```python
from build123d import *

# Parameters (mm, degrees)
F2_R     = 7.62
F3_DEPTH = 76.2


with BuildPart() as f1:
    # F0 (on Front) → F1 (revolve)
    with BuildSketch(Plane.XZ):
        with BuildLine():
            Line((0, -25.4), (0, 25.4))
            ThreePointArc((0, 25.4), (-25.4, 0), (0, -25.4))
        make_face()
    revolve(axis=Axis((0, 0, 0), (0, 0, -1)))

    # F2 (on Front) → F3 (cut)
    with BuildSketch(Plane.XZ):
        with Locations((-11.303624, 9.141192)):
            Circle(F2_R)
        with Locations((10.320701, 9.534361)):
            Circle(F2_R)
        with Locations((9.141192, -12.483133)):
            Circle(F2_R)
        with Locations((-9.337776, -13.662642)):
            Circle(F2_R)
    extrude(amount=-F3_DEPTH, mode=Mode.SUBTRACT)


solid = f1.part
```
Check sheet for the modelled part. Datum: model origin and axes. Units: mm. Give positions to 0.01 mm unless a question says otherwise; leave off trailing zeros. Order: outer loops, then holes, each group sorted by start corner. A loop starts at its lowest first (then second) coordinate and runs counter-clockwise, first axis right, second up. Notation, with made-up numbers: M 64,7.25 L 118,7.25 A23 cw 118,25.25 Z; hole C 60,20.5 d2. An arc over 180 degrees is marked long. Answer in a Markdown table with one row per item. Add a question column.
Q1. Sectioned sample at D-D, the plane x = -8. Record the boundary of the cut face in (y, z), and give its area (3 significant figures).
Q2. Gauge pin test, flat ends, axial feed: pin 1 Ø17 at (x, z) = (-9, 11) entering from +Y; pin 2 Ø24.5 at (x, z) = (9.14, -12.48) entering from +Y; pin 3 Ø4.5 at (x, z) = (12, 8) entering from +Y. Record the tip position at first contact, or that the pin passes through.
Q3. Thickness scan on L1, parallel to X at y = 1.5, z = 13; L2, parallel to X at y = 6, z = 5; L3, parallel to Y at x = -3, z = 2. Record the ranges inside material, lowest first.
Q4. Sectioned sample at A-A, the plane y = 10. Record the boundary of the cut face in (x, z), and give its area (3 significant figures).
Q5. Sectioned sample at B-B, the plane z = 15.5. Record the boundary of the cut face in (x, y).
Q6. Sectioned sample at C-C, the plane y = 3. Record the boundary of the cut face in (x, z).
Verdict:
| question | item | result |
|---|---|---|
| 1 | outline | M 0,-21.16 L 0,-6.16 L 23.31,-6.16 A24.11 ccw 24,2.27 L 0,2.27 L 0,16.01 L 18.03,16.01 A24.11 ccw long 11.54,-21.16 Z |
| 1 | area | 1,240 mm² |
| 2 | pin 1 | y = 24.75 |
| 2 | pin 2 | y = 25.2 |
| 2 | pin 3 | y = 0 |
| 3 | L1 | -21.77 to -17.87, -4.73 to 3.53, 17.11 to 21.77 |
| 3 | L2 | -24.17 to -17.7, -4.91 to 4.2, 16.44 to 24.17 |
| 3 | L3 | -25.14 to 25.14 |
| 4 | outline | M -16.33,-16.69 A7.62 cw long -9.61,-21.28 A23.35 ccw long Z; hole C -11.3,9.14 d15.24; hole C 9.14,-12.48 d15.24; hole C 10.32,9.53 d15.24 |
| 4 | area | 988 mm² |
| 5 | outline | M -15.5,0 L -15.5,12.83 A20.12 ccw long 15.06,13.34 L 15.06,0 L 5.58,0 L 5.58,19.33 A20.12 ccw -7.1,18.83 L -7.1,0 Z |
| 6 | outline | C 0,0 d50.44; hole C -11.3,9.14 d15.24; hole C -9.34,-13.66 d15.24; hole C 9.14,-12.48 d15.24; hole C 10.32,9.53 d15.24 |
